from build123d import *

# Parameters (mm, degrees)
SKETCH1_R               = 50
BOSS_EXTRUDE1_DEPTH     = 300
CUT_EXTRUDE1_DEPTH      = 364.987490242
CUT_EXTRUDE1_DEPTH_BACK = 364.987490242
SKETCH4_W               = 12.597132099
SKETCH4_H               = 279.427293847
CUT_EXTRUDE2_DEPTH      = 364.987490242
CUT_EXTRUDE2_DEPTH_BACK = 364.987490242
SKETCH5_W               = 13.949781053
SKETCH5_H               = 363.760783887


with BuildPart() as part:
    # Sketch1 → Boss-Extrude1 (new body)
    with BuildSketch(Plane(origin=(0, 0, 0), x_dir=(1, 0, 0), z_dir=(0, 1, 0))):
        with Locations(Location((0, 0, 0), (0, 0, 270))):
            Circle(SKETCH1_R)
    extrude(amount=BOSS_EXTRUDE1_DEPTH)

    # Sketch2 → Revolve1 (revolve)
    with BuildSketch(Plane.XY):
        with BuildLine():
            Line((-36.526834234, 250), (-36.526834234, 350))
            ThreePointArc((-36.526834234, 350), (13.473165766, 300), (-36.526834234, 250))
        make_face()
    revolve(axis=Axis((-36.526834234, 250, 0), (0, 1, 0)))

    # Sketch3 → Revolve2 (revolve)
    with BuildSketch(Plane.XY):
        with BuildLine():
            Line((0, -50), (0, 50))
            ThreePointArc((0, 50), (50, 0), (0, -50))
        make_face()
    revolve(axis=Axis((0, -50, 0), (0, 1, 0)))

    # Sketch4 → Cut-Extrude1 (cut, two sides: drawn at the far end of the back side and taken through both)
    with BuildSketch(Plane.XY.offset(-CUT_EXTRUDE1_DEPTH_BACK)):
        with Locations((-53.478127305, 108.200425306)):
            Rectangle(SKETCH4_W, SKETCH4_H)
    extrude(amount=CUT_EXTRUDE1_DEPTH + CUT_EXTRUDE1_DEPTH_BACK, mode=Mode.SUBTRACT)

    # Sketch5 → Cut-Extrude2 (cut, two sides: drawn at the far end of the back side and taken through both)
    with BuildSketch(Plane(origin=(0, 0, 0), x_dir=(0, 0, -1), z_dir=(1, 0, 0)).offset(-CUT_EXTRUDE2_DEPTH_BACK)):
        with Locations((-51.783725954, 173.445822779)):
            Rectangle(SKETCH5_W, SKETCH5_H)
    extrude(amount=CUT_EXTRUDE2_DEPTH + CUT_EXTRUDE2_DEPTH_BACK, mode=Mode.SUBTRACT)


solid = part.part
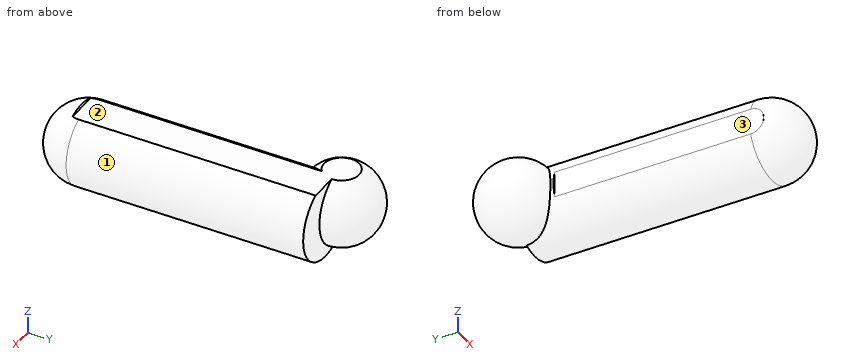
The listing builds one solid part. Answer for the finished solid, in the listing's coordinates (mm). Face numbers are marked on the shaded views. A direction names the side the tool comes from. Give positions to 0.01 mm unless a question says otherwise; leave off trailing zeros. Write each loop counter-clockwise with the first axis right and the second up, starting at its lowest first coordinate (ties: lowest second). Pieces come first, ordered by that corner, then holes. Notation, with made-up numbers: (12.25, -1.75) -> (23.25, -1.75) arc R22 ccw to (23.25, 20.25) -> close; hole circle Ø11 at (22.5, 50). An arc over 180 degrees is marked (long way). Use a Markdown table: item, result.
(1) Section B-B, the plane x = 0 is taken. Determine the outline of the cut face in (y, z).
Return value:
| item | result |
|---|---|
| outline | (-8.43, 44.81) -> (-8.43, 49.28) arc R50 ccw to (0, -50) -> (300, -50) -> (300, -34.14) arc R34.14 ccw to (300, 34.14) -> (300, 44.81) -> close |
(2) Flat-ended cylindrical pins translate along their axes: P1, Ø3, axis at x = -18, z = -15, coming from the -Y side; P2, Ø4, axis at y = 157, z = 13, coming from the +X side (3 decimals); P3, Ø3, axis at x = -49, z = -8, coming from the -Y side. Find the tip coordinate at first contact, or state that the pin passes through.
Return value:
| item | result |
|---|---|
| P1 | y = -44.93 |
| P2 | x = 48.775 |
| P3 | y = 247.91 |
(3) Section D-D, the plane x = -27 is taken. Determine the outline of the cut face in (y, z).
Return value:
| item | result |
|---|---|
| outline | (0, -42.08) -> (274.74, -42.08) arc R49.08 ccw (long way) to (320.04, 44.81) -> (279.96, 44.81) arc R49.08 ccw to (274.74, 42.08) -> (0, 42.08) arc R42.08 ccw to start |
(4) For the marked faces 1, 2 and 3, determine the directions among +Z, -Z, +X, -X, +Y, -Y from which every point of the face is accessible in a straight line to the end or side of a thin tool.
Return value:
| item | result |
|---|---|
| face 1 | -Y |
| face 2 | +Z, +X, -X, +Y |
| face 3 | +Z, -Z, -X, -Y |
(5) Find the intervals of material crossed by probe 1 along Y at (x, z) = (33, 31.5); probe 2 along Z at (x, y) = (30.5, 289); probe 3 along Z at (x, y) = (5, 316.5), in increasing order. Write a range as from..to.
Return value:
| item | result |
|---|---|
| probe 1 | -20.46..300 |
| probe 2 | -39.62..39.62 |
| probe 3 | -22.43..22.43 |
(6) Section C-C, the plane y = -25.5 is taken. Determine the outline of the cut face in (x, z), then the cut area to 3 significant figures.
Return value:
| item | result |
|---|---|
| outline | circle Ø86.02 at (0, 0) |
| area | 5,810 mm2 |
(7) Section A-A, the plane z = 0 is taken. Determine the outline of the cut face in (x, y), then the cut area to 3 significant figures.
Return value:
| item | result |
|---|---|
| outline | (-50, 247.91) -> (-47.18, 247.91) -> (-47.18, -16.56) arc R50 ccw to (50, 0) -> (50, 300) -> (13.47, 300) arc R50 ccw (long way) to (-50, 251.85) -> close |
| area | 38,400 mm2 |
